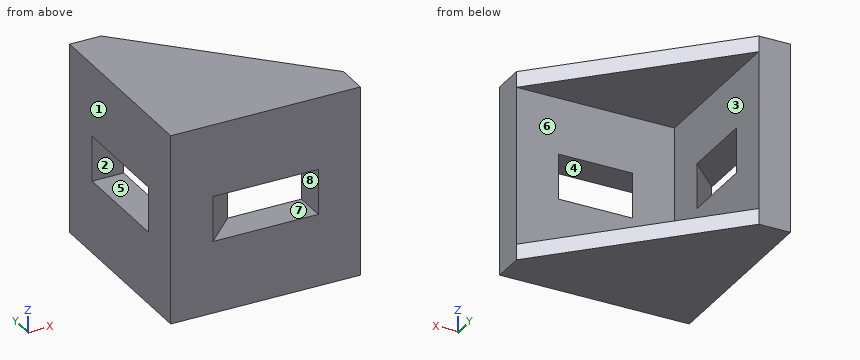
```python
from build123d import *

# Parameters (mm, degrees)
BOSS_EXTRUDE1_DEPTH = 9
CUT_EXTRUDE1_DEPTH  = 7.5
CUT_EXTRUDE2_DEPTH  = 2.15


with BuildPart() as part:
    # Sketch1 → Boss-Extrude1 (new, symmetric)
    with BuildSketch(Plane.XY):
        Polygon((0, 0), (0, 18), (3, 18), (18, 3), (18, 0), align=None)
    extrude(amount=BOSS_EXTRUDE1_DEPTH, both=True)

    # Sketch2 → Cut-Extrude1 (cut, symmetric)
    with BuildSketch(Plane.XY):
        Polygon((3, 18), (3, 3), (18, 3), align=None)
    extrude(amount=CUT_EXTRUDE1_DEPTH, both=True, mode=Mode.SUBTRACT)

    # Sketch3 → Cut-Extrude2 (cut, symmetric)
    with BuildSketch(Plane.XY):
        Polygon((0, 14), (3, 14), (3, 7), (0, 4), align=None)
        Polygon((7, 3), (14, 3), (14, 0), (4, 0), align=None)
    extrude(amount=CUT_EXTRUDE2_DEPTH, both=True, mode=Mode.SUBTRACT)


solid = part.part
```
Here's how the part is built. I have some questions about the finished solid (model axes, mm). Face numbers are marked on the shaded views. A direction names the side the tool comes from. Round coordinates to 2 decimals unless told otherwise and drop trailing zeros. Order: outer loops, then holes, each group sorted by start corner. A loop starts at its lowest first (then second) coordinate and runs counter-clockwise, first axis right, second up. Notation, with made-up numbers: M -36,55 L 18,55 A31 cw 18,85 Z; hole C -7,3.5 d7. An arc over 180 degrees is marked long. One line per question, with ' | ' between items.
1) I want a section at D-D, the plane x = 15.5. Write out the boundary of the cut face in (y, z).
Working result:
outline: M 0,-9 L 5.5,-9 L 5.5,-7.5 L 3,-7.5 L 3,7.5 L 5.5,7.5 L 5.5,9 L 0,9 Z
2) I want a section at C-C, the plane z = 0. Write out the boundary of the cut face in (x, y), then the cut area to 3 significant figures.
Working result:
outline: M 0,0 L 4,0 L 7,3 L 3,3 L 3,7 L 0,4 Z; M 0,14 L 3,14 L 3,18 L 0,18 Z; M 14,0 L 18,0 L 18,3 L 14,3 Z | area: 48.0 mm²
3) For pin 1 Ø7.5 at (x, z) = (11, 0) entering from +Y, with a flat end and sliding along its axis, tell me the tip position at first contact or that it passes through.
Working result:
pin 1: y = 3
4) For the marked faces 5, 6, 7 and 8, which set-ups out of +Z, -Z, +X, -X, +Y, -Y let a thin tool reach every point of the face, with its end or its side?
Working result:
face 5: -X | face 6: +X, +Y | face 7: -Y | face 8: +Y, -Y
5) I want a section at B-B, the plane y = 4.75. Write out the boundary of the cut face in (x, z), then the cut area to 3 significant figures.
Working result:
outline: M 0,-9 L 16.25,-9 L 16.25,-7.5 L 3,-7.5 L 3,7.5 L 16.25,7.5 L 16.25,9 L 0,9 L 0,2.15 L 0.75,2.15 L 0.75,-2.15 L 0,-2.15 Z | area: 90.5 mm²
6) I want a section at A-A, the plane x = 7.5. Write out the boundary of the cut face in (y, z), then the cut area to 3 significant figures.
Working result:
outline: M 0,-9 L 13.5,-9 L 13.5,-7.5 L 3,-7.5 L 3,-2.15 L 0,-2.15 Z; M 0,2.15 L 3,2.15 L 3,7.5 L 13.5,7.5 L 13.5,9 L 0,9 Z | area: 72.6 mm²
7) I need wall thicknesses on line 1 along Z through (x, y) = (12.5, 6); line 2 along Z through (x, y) = (1, 7.5); line 3 along X through (y, z) = (9, 3.75). Which ranges of each line are inside material? Lowest first, please.
Working result:
line 1: -9 to -7.5, 7.5 to 9 | line 2: -9 to -2.15, 2.15 to 9 | line 3: 0 to 3
8) If we mould it in two halves opening along X, with no side actions, what happens to the marked faces 1, 2, 3 and 4? For each: +X half, -X half, draft (parallel to the pull), parting line (faces both ways), or undercut.
Working result:
face 1: -X half | face 2: draft | face 3: +X half | face 4: undercut
